Here's how the part is built. I have some questions about the finished solid (model axes, mm). Round coordinates to 2 decimals unless told otherwise and drop trailing zeros. Write each loop counter-clockwise with the first axis right and the second up, starting at its lowest first coordinate (ties: lowest second). Pieces come first, ordered by that corner, then holes. Notation, with made-up numbers: M 82,-7.75 L 86,-7.75 A18 cw 86,0.25 Z; hole C 48.5,50 d7. An arc over 180 degrees is marked long. Write item = value, one per line. Start each with the question number.
(1) I want a section at C-C (z = 1.4). List the corners of the cut face in (x, y) for me, and give its area (3 significant figures).
(2) I want a section at B-B (y = 21.75). List the corners of the cut face in (x, z) for me.
(3) I want a section at A-A (x = 22). List the corners of the cut face in (y, z) for me, and give its area (3 significant figures).
(4) I need wall thicknesses on line 1 along Y through (x, z) = (22, 1.9); line 2 along Y through (x, z) = (22, 4.6); line 3 along Z through (x, y) = (19, 25.25). Which ranges of each line are inside material? Lowest first, please.
(5) I want a section at D-D (y = 25.25). List the corners of the cut face in (x, z) for me, and give its area (3 significant figures).
```python
from build123d import *

# Parameters (mm, degrees)
F0_W     = 44
F0_H     = 28.6
F0_R     = 12
F1_DEPTH = 5
F0_R_2   = 9.5
F2_DEPTH = 3


with BuildPart() as f1:
    # F0 (on Top) → F1 (new body)
    with BuildSketch(Plane.XY):
        with Locations((22, 14.3)):
            Rectangle(F0_W, F0_H)
        with Locations((22, 14.3)):
            Circle(F0_R, mode=Mode.SUBTRACT)
    extrude(amount=F1_DEPTH)

    # F0 (on Top) → F2 (join)
    with BuildSketch(Plane.XY):
        with Locations((22, 14.3)):
            Circle(F0_R)
        with Locations((22, 14.3)):
            Circle(F0_R_2, mode=Mode.SUBTRACT)
    extrude(amount=F2_DEPTH)


solid = f1.part
```
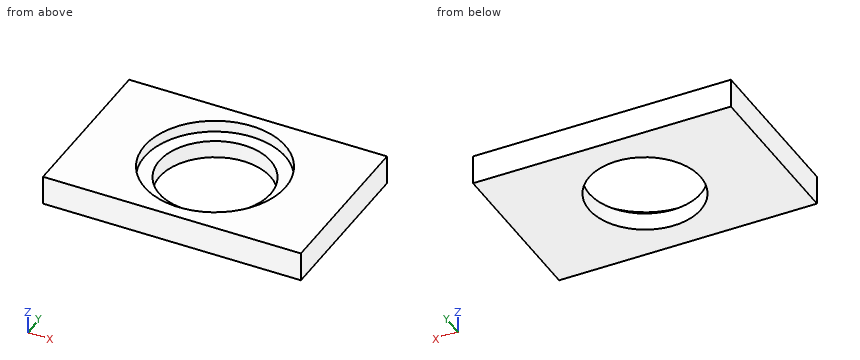
Returned:
q1.outline = M 0,0 L 44,0 L 44,28.6 L 0,28.6 Z; hole C 22,14.3 d19
q1.area = 975 mm²
q2.outline = M 0,0 L 16.11,0 L 16.11,3 L 12.59,3 L 12.59,5 L 0,5 Z; M 27.89,0 L 44,0 L 44,5 L 31.41,5 L 31.41,3 L 27.89,3 Z
q3.outline = M 0,0 L 4.8,0 L 4.8,3 L 2.3,3 L 2.3,5 L 0,5 Z; M 23.8,0 L 28.6,0 L 28.6,5 L 26.3,5 L 26.3,3 L 23.8,3 Z
q3.area = 38.0 mm²
q4.line_1 = 0 to 4.8, 23.8 to 28.6
q4.line_2 = 0 to 2.3, 26.3 to 28.6
q4.line_3 = 0 to 3
q5.outline = M 0,0 L 44,0 L 44,5 L 26.91,5 L 26.91,3 L 17.09,3 L 17.09,5 L 0,5 Z
q5.area = 200 mm²
